Autodesk Fusion 360 part; units mm, degrees
box "BoxPrimitive1" add length 89 width 100 height 2 placed x (0, 0, 1) y (1, 0, 0) z (0, 1, 0) at (0, 0, 0)
box "BoxPrimitive2" add length 89 width 2 height 7 placed x (0, 0, 1) y (1, 0, 0) z (0, 1, 0) at (0, 2, 0)
box "BoxPrimitive3" add length 89 width 2 height 7 placed x (0, 0, 1) y (1, 0, 0) z (0, 1, 0) at (98, 2, 0)
box "BoxPrimitive4" add length 2 width 96 height 7 placed x (0, 0, 1) y (1, 0, 0) z (0, 1, 0) at (2, 2, 0)
box "BoxPrimitive5" add length 2 width 96 height 7 placed x (0, 0, -1) y (-1, 0, 0) z (0, 1, 0) at (98, 2, 89)
box "BoxPrimitive6" cut length 7 width 13 height -2 placed x (0, 0, -1) y (-1, 0, 0) z (0, 1, 0) at (25, 2, 19)
Here's how the part is built. I have some questions about the finished solid (model axes, mm). A direction names the side the tool comes from. Give positions to 0.01 mm unless a question says otherwise; leave off trailing zeros. Write each loop counter-clockwise with the first axis right and the second up, starting at its lowest first coordinate (ties: lowest second). Pieces come first, ordered by that corner, then holes.
(1) Thinking about a two-plate mould opening in Z: for faces 3 (the face through (51, 4, 89)), 4 (the face through (2, 5, 45)), 5 (the face through (100, 4, 45)), 6 (the face through (51, 2, 44)), which applies, pulls with the +Z half, pulls with the -Z half, needs draft (parallel to the pull), parting line crosses it, or undercut?
Output values:
face 3: pulls with the +Z half
face 4: undercut
face 5: needs draft
face 6: undercut
(2) Will this pin go through, and if not, where does the flat tip stop? pin 1 (2 mm diameter, centred on x = 88.5, z = 50.5, fed in from +Y).
Output values:
pin 1: stops at y = 2
(3) If I drill on L1, parallel to X at y = 3, z = 12; L2, parallel to Z at x = 26.5, y = 6.5; L3, parallel to Y at x = 49.5, z = 45.5, over which ranges is the centre line in solid material (lowest first)?
Output values:
L1: x = 0 to 2, 98 to 100
L2: z = 0 to 2, 87 to 89
L3: y = 0 to 2
(4) Imagine slicing it at C-C, the plane x = 59. Write out the boundary of the cut face in (y, z).
Output values:
outline: (0, 0) - (9, 0) - (9, 2) - (2, 2) - (2, 87) - (9, 87) - (9, 89) - (0, 89) - close
(5) On a 3-axis mill with a long thin cutter (end or side, diameter ignored), from which of +Z, -Z, +X, -X, +Y, -Y can I reach the whole of each face in a straight line? I mean faces 1 (the face through (0, 4, 45)), 2 (the face through (49, 5, 2)). Say none if no direction works.
Output values:
face 1: +Z, -Z, -X, +Y, -Y
face 2: +Y
(6) Imagine slicing it at B-B, the plane y = 5. Write out the boundary of the cut face in (x, z).
Output values:
outline: (0, 0) - (100, 0) - (100, 89) - (0, 89) - close; hole (2, 2) - (98, 2) - (98, 87) - (2, 87) - close
(7) Imagine slicing it at A-A, the plane z = 13.5. Write out the boundary of the cut face in (x, y).
Output values:
outline: (0, 0) - (12, 0) - (12, 2) - (2, 2) - (2, 9) - (0, 9) - close; (25, 0) - (100, 0) - (100, 9) - (98, 9) - (98, 2) - (25, 2) - close
